Design review of the part built by this model. Coordinates are the model's own, in mm. Round coordinates to 2 decimals unless told otherwise and drop trailing zeros. Write each loop counter-clockwise with the first axis right and the second up, starting at its lowest first coordinate (ties: lowest second). Pieces come first, ordered by that corner, then holes.
from build123d import *

# Parameters (mm, degrees)
SKETCH_1_W          = 40
SKETCH_1_H          = 15
EXTRUDE_1_DEPTH     = 6
SKETCH_2_R          = 2.5
CUT_EXTRUDE_1_DEPTH = 23.186707732
FILLET_1_R          = 3


with BuildPart() as part:
    # 草图1 → 凸台-拉伸1 (new body)
    with BuildSketch(Plane.XY):
        Rectangle(SKETCH_1_W, SKETCH_1_H)
    extrude(amount=EXTRUDE_1_DEPTH)

    # 草图2 → 切除-拉伸1 (cut, through all)
    with BuildSketch(Plane.XY.offset(6)):
        with Locations((-12.5, 0)):
            Circle(SKETCH_2_R)
        with Locations(Location((12.5, 0, 0), (0, 0, 180))):
            Circle(SKETCH_2_R)
    extrude(amount=-CUT_EXTRUDE_1_DEPTH, mode=Mode.SUBTRACT)

    # 圆角1
    fillet_1_edges = [part.edges().sort_by_distance(p)[0] for p in [
        (20, -7.5, 3),
        (-20, -7.5, 3),
        (-20, 7.5, 3),
        (20, 7.5, 3),
    ]]
    fillet(fillet_1_edges, radius=FILLET_1_R)


solid = part.part
1) Add section B-B on y = 0. State the section outline as (x, z) points, and give its area (3 significant figures).
2) Add section C-C on z = 3.05. State the section outline as (x, y) points, and give its area (3 significant figures).
3) Add section A-A on x = 12.5. State the section outline as (y, z) points.
4) For P1, Ø2, axis at y = -6, z = 3.5, coming from the +X side, flat-tipped, find the tip position at first contact; note if it passes through.
5) Add section D-D on x = -11.5. State the section outline as (y, z) points.
6) The part is to be moulded in two halves that separate along X. For faces 1 (the face through (0, 0, 0)), 2 (the face through (-20, 0, 3)), 3 (the face through (-15, 0, 3)), say which applies: pulls with the +X half, pulls with the -X half, needs draft (parallel to the pull), parting line crosses it, or undercut.
7) For line 1 along Y through (x, z) = (12.5, 2.95); line 2 along X through (y, z) = (1.25, 0.65); line 3 along X through (y, z) = (-2.25, 2.1), list the stretches that pass through material, from the lowest coordinate up.
Computed:
1. outline: (-20, 0) - (-15, 0) - (-15, 6) - (-20, 6) - close; (-10, 0) - (10, 0) - (10, 6) - (-10, 6) - close; (15, 0) - (20, 0) - (20, 6) - (15, 6) - close
1. area: 180 mm2
2. outline: (-20, -4.5) arc R3 ccw to (-17, -7.5) - (17, -7.5) arc R3 ccw to (20, -4.5) - (20, 4.5) arc R3 ccw to (17, 7.5) - (-17, 7.5) arc R3 ccw to (-20, 4.5) - close; hole circle Ø5 at (-12.5, 0); hole circle Ø5 at (12.5, 0)
2. area: 553 mm2
3. outline: (-7.5, 0) - (-2.5, 0) - (-2.5, 6) - (-7.5, 6) - close; (2.5, 0) - (7.5, 0) - (7.5, 6) - (2.5, 6) - close
4. P1: stops at x = 19.96
5. outline: (-7.5, 0) - (-2.29, 0) - (-2.29, 6) - (-7.5, 6) - close; (2.29, 0) - (7.5, 0) - (7.5, 6) - (2.29, 6) - close
6. face 1: needs draft
6. face 2: pulls with the -X half
6. face 3: undercut
7. line 1: y = -7.5 to -2.5, 2.5 to 7.5
7. line 2: x = -20 to -14.67, -10.33 to 10.33, 14.67 to 20
7. line 3: x = -20 to -13.59, -11.41 to 11.41, 13.59 to 20
